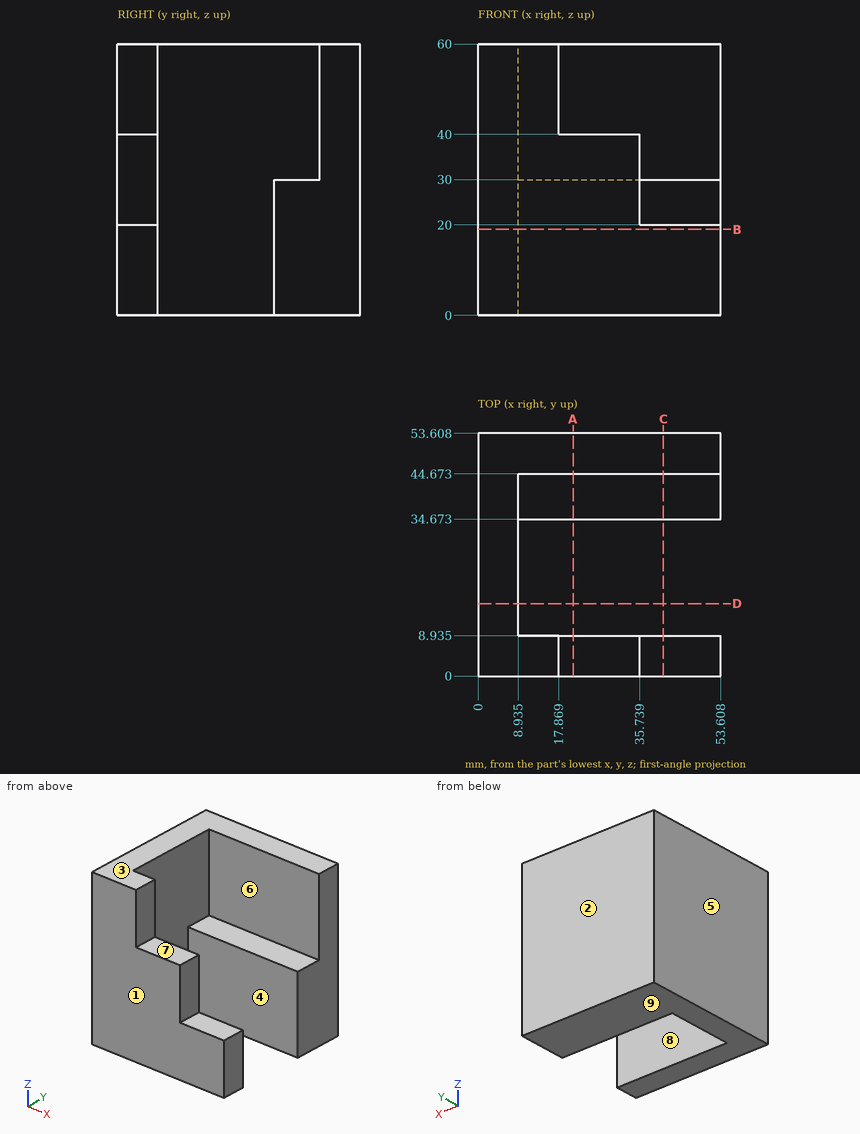
Here's the drawing with two shaded views (mm, measured from the low corner). I have some questions. A direction names the side the tool comes from. Give positions to 0.01 mm unless a question says otherwise; leave off trailing zeros. Order: outer loops, then holes, each group sorted by start corner. A loop starts at its lowest first (then second) coordinate and runs counter-clockwise, first axis right, second up. Notation, with made-up numbers: (68, 86.5) -> (98, 86.5) arc R17 ccw to (98, 97.5) -> close; hole circle Ø8 at (85, 3.5). An arc over 180 degrees is marked (long way). One line per item, written item: value. Start each with the question number.
1. Imagine slicing it at B-B, the plane z = 19. List the corners of the cut face in (x, y) for me (1 decimal), plus the area to 3 significant figures.
2. Will these pins go through, and if not, where does the flat tip stop? pin 1 Ø18 at (y, z) = (31.5, 42.5) entering from +X (1 decimal); pin 2 Ø8 at (x, y) = (31.5, 39.5) entering from +Z; pin 3 Ø10 at (y, z) = (6.5, 30) entering from +X; pin 4 Ø12 at (x, y) = (22, 20.5) entering from -Z.
3. For the marked faces 5, 6, 7, 8 and 9, which set-ups out of +Z, -Z, +X, -X, +Y, -Y let a thin tool reach every point of the face, with its end or its side?
4. I need wall thicknesses on probe 1 along Y at (x, z) = (15.5, 5) (1 decimal); probe 2 along Y at (x, z) = (28.5, 39) (1 decimal); probe 3 along X at (y, z) = (26, 53.5) (1 decimal). Which ranges of each line are inside material? Lowest first, please. Write a range as from..to.
5. Imagine slicing it at D-D, the plane y = 16. List the corners of the cut face in (x, z) for me (1 decimal), plus the area to 3 significant figures.
6. Imagine slicing it at A-A, the plane x = 21. List the corners of the cut face in (y, z) for me (1 decimal), plus the area to 3 significant figures.
7. We'd pull the mould along Y, two halves only. Please class the marked faces 1, 2, 3 and 4: released by +Y, released by -Y, zero draft, split by the parting line, or undercut.
8. Imagine slicing it at C-C, the plane x = 41. List the corners of the cut face in (y, z) for me (1 decimal).
Values follow:
1. outline: (0, 0) -> (53.6, 0) -> (53.6, 8.9) -> (8.9, 8.9) -> (8.9, 34.7) -> (53.6, 34.7) -> (53.6, 53.6) -> (0, 53.6) -> close
1. area: 1,720 mm2
2. pin 1: stops at x = 8.9
2. pin 2: stops at z = 30
2. pin 3: stops at x = 35.74
2. pin 4: passes through
3. face 5: +Z, -Z, -X, +Y, -Y
3. face 6: +Z, +X
3. face 7: +Z, +X, -Y
3. face 8: +Z, -Z, +X
3. face 9: -Z, +X, -X, +Y, -Y
4. probe 1: y = 0..8.9, 34.7..53.6
4. probe 2: y = 0..8.9, 44.7..53.6
4. probe 3: x = 0..8.9
5. outline: (0, 0) -> (8.9, 0) -> (8.9, 60) -> (0, 60) -> close
5. area: 536 mm2
6. outline: (0, 0) -> (8.9, 0) -> (8.9, 40) -> (0, 40) -> close; (34.7, 0) -> (53.6, 0) -> (53.6, 60) -> (44.7, 60) -> (44.7, 30) -> (34.7, 30) -> close
6. area: 1,190 mm2
7. face 1: released by -Y
7. face 2: released by +Y
7. face 3: zero draft
7. face 4: undercut
8. outline: (0, 0) -> (8.9, 0) -> (8.9, 20) -> (0, 20) -> close; (34.7, 0) -> (53.6, 0) -> (53.6, 60) -> (44.7, 60) -> (44.7, 30) -> (34.7, 30) -> close
